Geometry check sheet. Reference: the model listing, model coordinates, mm. A direction names the side the tool comes from. Coordinates: 2 decimals unless noted, no trailing zeros. Loops run counter-clockwise (first coordinate to the right, second up) from the corner with the lowest first, then second, coordinate; pieces in that order, holes last.
from build123d import *

# Parameters (mm, degrees)
BOSS_EXTRUDE1_DEPTH = 1.6
SKETCH1_R           = 4.985014332
BOSS_EXTRUDE2_DEPTH = 5.5


with BuildPart() as part:
    # Board_Outline → Boss-Extrude1 (new body)
    with BuildSketch(Plane.XY):
        Polygon((0, 12.192), (0, 1.905), (0.064911, 1.41195), (0.255222, 0.9525), (0.557962, 0.557962), (0.9525, 0.255222), (1.41195, 0.064911), (1.905, 0), (23.495, 0), (23.98805, 0.064911), (24.4475, 0.255222), (24.842038, 0.557962), (25.142046405, 0.948978179), (25.325809203, 1.389546655), (25.4, 1.884780797), (25.4, 1.905), (25.4, 12.192), (25.335089, 12.68505), (25.144778, 13.1445), (24.842038, 13.539038), (24.4475, 13.841778), (23.98805, 14.032089), (23.495, 14.097), (1.905, 14.097), (1.41195, 14.032089), (0.9525, 13.841778), (0.557962, 13.539038), (0.255222, 13.1445), (0.064911, 12.68505), align=None)
    extrude(amount=BOSS_EXTRUDE1_DEPTH)

    # Sketch1 → Boss-Extrude2 (add)
    with BuildSketch(Plane(origin=(0, 0, 0), x_dir=(-1, 0, 0), z_dir=(0, 0, -1))):
        with Locations(Location((-18.349836539, 7.101234384, 0), (0, 0, 180))):
            Circle(SKETCH1_R)
    extrude(amount=BOSS_EXTRUDE2_DEPTH)


solid = part.part
1) Section check B-B on x = 14.25. Record the cut outline in (y, z), and give its area (3 significant figures).
Data:
outline: (0, 0) - (4.27, 0) - (4.27, -5.5) - (9.94, -5.5) - (9.94, 0) - (14.1, 0) - (14.1, 1.6) - (0, 1.6) - close
area: 53.7 mm2
2) Section check C-C on z = -2.75. Record the cut outline in (x, y), and give its area (3 significant figures).
Data:
outline: circle Ø9.97 at (18.35, 7.1)
area: 78.1 mm2
3) Material ranges on probe 1 along Z at (x, y) = (5, 13.25); probe 2 along Y at (x, z) = (18.5, -5); probe 3 along X at (y, z) = (4.5, -1.75), recorded low to high.
Data:
probe 1: z = 0 to 1.6
probe 2: y = 2.12 to 12.08
probe 3: x = 14.1 to 22.6
4) Access from +Z, -Z, +X, -X, +Y, -Y to the whole of each face (thin tool, end or side, straight path). Record for faces 1 (the flat face through (25.4, 7, 1)), 2 (the cylindrical face through (23.105, 5.604, -2.712)).
Data:
face 1: +Z, -Z, +X, +Y, -Y
face 2: -Z
5) Depth check by flat-ended pin: pin 1 (4 mm diameter, centred on x = 8.5, y = 2.5, fed in from -Z); pin 2 (1 mm diameter, centred on y = 4, z = -3, fed in from -X); pin 3 (4 mm diameter, centred on y = 7, z = -3, fed in from -X). Enter the tip coordinate at first touch or a pass-through.
Data:
pin 1: stops at z = 0
pin 2: stops at x = 14.1
pin 3: stops at x = 13.36
6) Section check A-A on y = 9. Record the cut outline in (x, z), and give its area (3 significant figures).
Data:
outline: (0, 0) - (13.74, 0) - (13.74, -5.5) - (22.96, -5.5) - (22.96, 0) - (25.4, 0) - (25.4, 1.6) - (0, 1.6) - close
area: 91.3 mm2
